Check sheet for the modelled part. Datum: model origin and axes. Units: mm. Face numbers are marked on the shaded views. A direction names the side the tool comes from. Coordinates: 2 decimals unless noted, no trailing zeros. Write each loop counter-clockwise with the first axis right and the second up, starting at its lowest first coordinate (ties: lowest second). Pieces come first, ordered by that corner, then holes. Notation, with made-up numbers: (-21.5, 28) -> (-0.5, 28) arc R13 cw to (-0.5, 43) -> close; hole circle Ø5 at (-28.75, 80.25). An arc over 180 degrees is marked (long way). One line per item, written item: value. Start each with the question number.
1) Sectioned sample at B-B on x = 0. Enter the section's corners in (y, z) (3 decimals).
2) Gauge pin test, flat ends, axial feed: P1, Ø0.7, axis at y = 11.5, z = -9.5, coming from the -X side; P2, Ø4, axis at y = 20.5, z = 19.5, coming from the +X side; P3, Ø8, axis at y = 3, z = 11.5, coming from the +X side; P4, Ø1, axis at y = 9.5, z = 21, coming from the +X side (3 decimals). Record the tip position at first contact, or that the pin passes through.
3) Scan lines: line 1 along Y through (x, z) = (0, 40); line 2 along Y through (x, z) = (-10, 34.5); line 3 along Z through (x, y) = (-12.75, 7.25). Record each from-to range of solid material in increasing order. Write a range as [from, to].
4) Sectioned sample at A-A on z = -7.5. Enter the section's corners in (x, y).
5) Sectioned sample at C-C on y = 12.5. Enter the section's corners in (x, z).
6) Draft check along Y on the marked faces 4, 5, 6 and 7. Enter one of: +Y half, -Y half, draft (parallel to the pull), parting line (faces both ways), or undercut.
7) Set-up check for the marked faces 1, 2 and 3: record each of +Z, -Z, +X, -X, +Y, -Y from which the full face is reachable in a straight line by a thin tool's end or side.
8) Sectioned sample at D-D on x = -6. Enter the section's corners in (y, z).
```python
from build123d import *

# Parameters (mm, degrees)
SKETCH1_R           = 2.875
BOSS_EXTRUDE1_DEPTH = 20
SKETCH2_R           = 2.875
BOSS_EXTRUDE2_DEPTH = 14.99
BOSS_EXTRUDE3_DEPTH = 14.99
SKETCH4_R           = 14.125
SKETCH4_W           = 15
SKETCH4_H           = 14.99
SKETCH4_H_2         = 7.495
BOSS_EXTRUDE4_DEPTH = 6.25
SKETCH5_R           = 14.125
SKETCH5_R_2         = 12.625
BOSS_EXTRUDE5_DEPTH = 26
BOSS_EXTRUDE8_DEPTH = 14.99
CUT_EXTRUDE3_DEPTH  = 59.732465681


with BuildPart() as part:
    # Sketch1 → Boss-Extrude1 (new body)
    with BuildSketch(Plane(origin=(0, 0, 0), x_dir=(1, 0, 0), z_dir=(0, 1, 0))):
        with Locations(Location((0, 0, 0), (0, 0, 270))):
            Circle(SKETCH1_R)
    extrude(amount=BOSS_EXTRUDE1_DEPTH)

    # Sketch2 → Boss-Extrude2 (add)
    with BuildSketch(Plane(origin=(0, 2.5, 0), x_dir=(-1, 0, 0), z_dir=(0, -1, 0))):
        with BuildLine():
            Line((-4, 7.5), (-4, 10))
            ThreePointArc((-4, 10), (-5.75, 11.75), (-7.5, 10))
            Line((-7.5, 10), (-7.5, 0))
            ThreePointArc((-7.5, 0), (0, -7.5), (7.5, 0))
            Line((7.5, 0), (7.5, 10))
            ThreePointArc((7.5, 10), (5.75, 11.75), (4, 10))
            Line((4, 10), (4, 7.5))
            ThreePointArc((4, 7.5), (0, 3.5), (-4, 7.5))
        make_face()
        with Locations(Location((0, 0, 0), (0, 0, 90))):
            Circle(SKETCH2_R, mode=Mode.SUBTRACT)
    extrude(amount=-BOSS_EXTRUDE2_DEPTH)

    # Sketch3 → Boss-Extrude3 (add)
    with BuildSketch(Plane(origin=(0, 2.5, 0), x_dir=(-1, 0, 0), z_dir=(0, -1, 0))):
        with BuildLine():
            Line((7.5, 0), (7.5, -20.5))
            Line((7.5, -20.5), (-7.5, -20.5))
            Line((-7.5, -20.5), (-7.5, 0))
            ThreePointArc((-7.5, 0), (0, -7.5), (7.5, 0))
        make_face()
    extrude(amount=-BOSS_EXTRUDE3_DEPTH)

    # Sketch4 → Boss-Extrude4 (add)
    # profile 1 of 3: a face of its own
    with BuildSketch(Plane.XY.offset(20.5)):
        with Locations((0, 9.995)):
            Circle(SKETCH4_R)
        with Locations((0, 9.995)):
            Rectangle(SKETCH4_W, SKETCH4_H, mode=Mode.SUBTRACT)
    # profile 2 of 3: a face of its own
    with BuildSketch(Plane.XY.offset(20.5)):
        with Locations((0, 13.7425)):
            Rectangle(SKETCH4_W, SKETCH4_H_2)
    # profile 3 of 3: a face of its own
    with BuildSketch(Plane.XY.offset(20.5)):
        with Locations((0, 6.2475)):
            Rectangle(SKETCH4_W, SKETCH4_H_2)
    extrude(amount=BOSS_EXTRUDE4_DEPTH)

    # Sketch5 → Boss-Extrude5 (add)
    with BuildSketch(Plane.XY.offset(26.75)):
        with Locations((0, 9.995)):
            Circle(SKETCH5_R)
        with Locations(Location((0, 9.995, 0), (0, 0, 180))):
            Circle(SKETCH5_R_2, mode=Mode.SUBTRACT)
    extrude(amount=BOSS_EXTRUDE5_DEPTH)

    # Sketch6 → Boss-Extrude8 (add)
    with BuildSketch(Plane(origin=(0, 2.5, 0), x_dir=(-1, 0, 0), z_dir=(0, -1, 0))):
        with BuildLine():
            Line((-2.135439924, 16.706507736), (-5.67097383, 13.17097383))
            ThreePointArc((-5.67097383, 13.17097383), (-6.629279887, 12.013594636), (-7.354872555, 10.697770796))
            ThreePointArc((-7.354872555, 10.697770796), (-5.393648327, 11.713334026), (-4, 10))
            Line((-4, 10), (-4, 7.5))
            ThreePointArc((-4, 7.5), (-0.388580969, 3.518919138), (3.924502415, 6.726513871))
            Line((3.924502415, 6.726513871), (2.348994272, 5.151005728))
            ThreePointArc((2.348994272, 5.151005728), (-2.348994272, 5.151005728), (-2.348994272, 9.848994272))
            Line((-2.348994272, 9.848994272), (1.186539634, 13.384528178))
            ThreePointArc((1.186539634, 13.384528178), (1.186539634, 16.706507736), (-2.135439924, 16.706507736))
        make_face()
        with BuildLine():
            ThreePointArc((-7.5, 10), (-7.463334026, 10.356351673), (-7.354872555, 10.697770796))
            ThreePointArc((-7.354872555, 10.697770796), (-8.017652884, 7.692692975), (-7.5, 4.659245108))
            Line((-7.5, 4.659245108), (-7.5, 10))
        make_face()
        with BuildLine():
            Line((7.5, 9.375108987), (7.5, 4.675990723))
            ThreePointArc((7.5, 4.675990723), (9.895517957, 7.025549855), (7.5, 9.375108987))
        make_face()
    extrude(amount=-BOSS_EXTRUDE8_DEPTH)

    # Sketch7 → Cut-Extrude3 (cut, through all)
    with BuildSketch(Plane(origin=(0, 2.5, 0), x_dir=(-1, 0, 0), z_dir=(0, -1, 0))):
        Polygon((3.924502415, 6.726513871), (1.023758885, 9.627257401), (6.777821546, 15.381320062), (9.647679203, 12.449690659), align=None)
    extrude(amount=-CUT_EXTRUDE3_DEPTH, mode=Mode.SUBTRACT)


solid = part.part
```
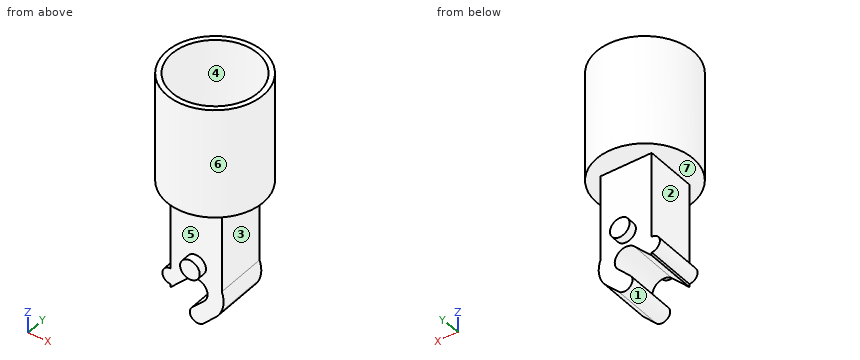
Answers:
1. outline: (-4.13, 20.5) -> (2.5, 20.5) -> (2.5, 2.875) -> (0, 2.875) -> (0, -2.875) -> (2.5, -2.875) -> (2.5, -4.178) -> (17.49, -4.178) -> (17.49, -2.875) -> (20, -2.875) -> (20, 2.875) -> (17.49, 2.875) -> (17.49, 20.5) -> (24.12, 20.5) -> (24.12, 52.75) -> (22.62, 52.75) -> (22.62, 26.75) -> (-2.63, 26.75) -> (-2.63, 52.75) -> (-4.13, 52.75) -> close; (2.5, -17.346) -> (17.49, -17.346) -> (17.49, -12.198) -> (2.5, -12.198) -> close
2. P1: stops at x = -8.55
2. P2: stops at x = 11.07
2. P3: stops at x = 7.5
2. P4: stops at x = 14.125
3. line 1: y = [-4.13, -2.63], [22.62, 24.12]
3. line 2: y = [0.02, 2.29], [17.7, 19.97]
3. line 3: z = [20.5, 52.75]
4. outline: (-9.85, 2.5) -> (-4.7, 2.5) -> (-4.7, 17.49) -> (-9.85, 17.49) -> close; (3.32, 2.5) -> (8.02, 2.5) -> (8.02, 17.49) -> (3.32, 17.49) -> close
5. outline: (-13.9, 20.5) -> (-7.5, 20.5) -> (-7.5, -4.68) arc R2.35 ccw (long way) to (-7.5, -9.38) -> (-7.5, -10) arc R1.75 ccw to (-7.48, -10.28) -> (-2.35, -5.15) arc R3.32 cw to (2.35, -9.85) -> (-1.19, -13.38) arc R2.35 ccw to (2.14, -16.71) -> (5.67, -13.17) arc R8.02 ccw to (7.5, -4.66) -> (7.5, 20.5) -> (13.9, 20.5) -> (13.9, 52.75) -> (12.37, 52.75) -> (12.37, 26.75) -> (-12.37, 26.75) -> (-12.37, 52.75) -> (-13.9, 52.75) -> close
6. face 4: undercut
6. face 5: -Y half
6. face 6: parting line
6. face 7: draft
7. face 1: +Y, -Y
7. face 2: -X, +Y, -Y
7. face 3: +X, +Y, -Y
8. outline: (-2.79, 20.5) -> (2.5, 20.5) -> (2.5, -8.8) -> (17.49, -8.8) -> (17.49, 20.5) -> (22.78, 20.5) -> (22.78, 52.75) -> (21.1, 52.75) -> (21.1, 26.75) -> (-1.11, 26.75) -> (-1.11, 52.75) -> (-2.79, 52.75) -> close
